Build history of the part. All positions in model axes, mm. Face numbers are marked on the shaded views. A direction names the side the tool comes from. Give positions to 0.01 mm unless a question says otherwise; leave off trailing zeros. Write each loop counter-clockwise with the first axis right and the second up, starting at its lowest first coordinate (ties: lowest second). Pieces come first, ordered by that corner, then holes. Notation, with made-up numbers: M -24.5,71 L 13.5,71 A25 cw 13.5,100 Z; hole C 52,9.5 d2. An arc over 180 degrees is marked long. Return JSON: item names as keys, results as strings. Group by question number.
Q1. Band-saw the part on A-A, the plane x = 0. Give the cut face in (y, z).
Q2. Pull direction X, two halves, no side cores. Call the marked faces 1, 2, 3 and 4: +X half, -X half, draft (parallel to the pull), parting line (faces both ways), or undercut.
Q3. Band-saw the part on C-C, the plane y = 2.8. Give the cut face in (x, z), then the cut area to 3 significant figures.
Q4. Band-saw the part on B-B, the plane z = 0. Give the cut face in (x, y), then the cut area to 3 significant figures.
Q5. Tool access for the marked faces 5, 6 and 7: list every direction of +Z, -Z, +X, -X, +Y, -Y with a clear straight run to the whole face (end or side of a thin tool).
Q6. Flat gauge pins, fed straight in: pin 1 Ø3 at (x, z) = (10, -10) entering from -Y; pin 2 Ø2.5 at (y, z) = (3, 0) entering from -X; pin 3 Ø1.5 at (x, y) = (-8.5, 4) entering from -Z. Where does each tip first touch, or does it go through?
Q7. Wall check: probe 1 along X at (y, z) = (3.25, 0); probe 2 along X at (y, z) = (0.4, 0). Give the ranges that are in metal, low to high.
Q8. Band-saw the part on D-D, the plane y = 0.9. Give the cut face in (x, z).
from build123d import *

# Parameters (mm, degrees)
CUT_EXTRUDE1_DEPTH = 19.936208702


with BuildPart() as part:
    # Sketch1 → Revolve1 (revolve)
    with BuildSketch(Plane.XY, mode=Mode.PRIVATE) as revolve1_sk:
        Polygon((-12.7, 2), (-11, 2), (-11, 0), (-9.7, 0), (-9.7, 2), (-7.5, 2), (-7.5, 6), (-10.7, 6), (-10.7, 3.143703987), (-12.7, 3.143703987), align=None)
        Polygon((-12.7, 3.143703987), (-10.7, 6), (-10.7, 3.143703987), align=None)
    revolve(revolve1_sk.sketch.rotate(Axis((0, 0, 0), (0, 1, 0)), 270), axis=Axis((0, 0, 0), (0, 1, 0)))

    # Sketch2 → Cut-Extrude1 (cut, through all)
    with BuildSketch(Plane(origin=(0, 0, 0), x_dir=(1, 0, 0), z_dir=(0, 1, 0))):
        with BuildLine():
            Line((-11.5, -1.5), (-11.5, 1.5))
            Line((-11.5, 1.5), (-12.611106216, 1.5))
            ThreePointArc((-12.611106216, 1.5), (-12.7, 0), (-12.611106216, -1.5))
            Line((-12.611106216, -1.5), (-11.5, -1.5))
        make_face()
        with BuildLine():
            ThreePointArc((12.7, 0), (12.677757076, 0.751315863), (12.611106216, 1.5))
            Line((12.611106216, 1.5), (11.5, 1.5))
            Line((11.5, 1.5), (11.5, -1.5))
            Line((11.5, -1.5), (12.611106216, -1.5))
            ThreePointArc((12.611106216, -1.5), (12.677757076, -0.751315863), (12.7, 0))
        make_face()
    extrude(amount=CUT_EXTRUDE1_DEPTH, mode=Mode.SUBTRACT)


solid = part.part
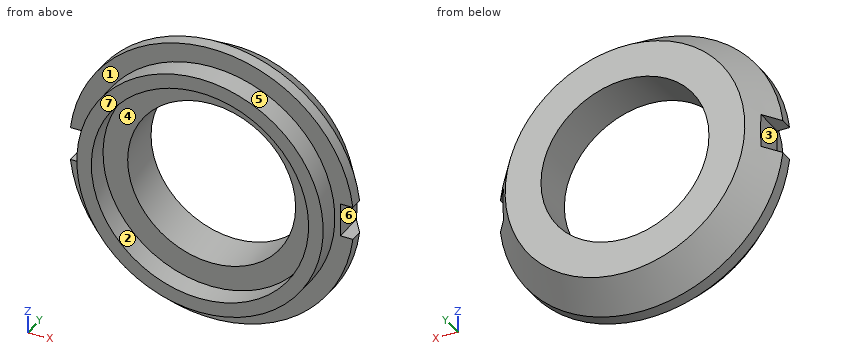
From the geometry:
{
 "1": {"outline": "M 0,-11 L 2,-11 L 2,-12.7 L 3.14,-12.7 L 6,-10.7 L 6,-7.5 L 2,-7.5 L 2,-9.7 L 0,-9.7 Z; M 0,9.7 L 2,9.7 L 2,7.5 L 6,7.5 L 6,10.7 L 3.14,12.7 L 2,12.7 L 2,11 L 0,11 Z"},
 "2": {"face 1": "draft", "face 2": "undercut", "face 3": "-X half", "face 4": "undercut"},
 "3": {"outline": "M -12.61,-1.5 A12.7 ccw 12.61,-1.5 L 11.5,-1.5 L 11.5,1.5 L 12.61,1.5 A12.7 ccw -12.61,1.5 L -11.5,1.5 L -11.5,-1.5 Z; hole C 0,0 d15", "area": "323 mm^2"},
 "4": {"outline": "M -11.5,2 L -11,2 L -11,0 L -9.7,0 L -9.7,2 L -7.5,2 L -7.5,6 L -10.7,6 L -11.5,4.86 Z; M 7.5,2 L 9.7,2 L 9.7,0 L 11,0 L 11,2 L 11.5,2 L 11.5,4.86 L 10.7,6 L 7.5,6 Z", "area": "36.3 mm^2"},
 "5": {"face 5": "-Y", "face 6": "+X, +Y, -Y", "face 7": "+Z, -Z, +X, -X, -Y"},
 "6": {"pin 1": "stops at y = 2", "pin 2": "stops at x = -11.5", "pin 3": "stops at z = -9.59"},
 "7": {"probe 1": "x = -11.5 to -7.5, 7.5 to 11.5", "probe 2": "x = -11 to -9.7, 9.7 to 11"},
 "8": {"outline": "C 0,0 d22; hole C 0,0 d19.4"}
}
